Autodesk Inventor part; units mm, degrees
ref_plane "YZ Plane" through (0, 0, 0) normal (1, 0, 0) x (0, 1, 0)
ref_plane "XZ Plane" through (0, 0, 0) normal (0, 1, 0) x (-1, 0, 0)
ref_plane "XY Plane" through (0, 0, 0) normal (0, 0, 1) x (1, 0, 0)
sketch "Sketch2" plane through (0, 0, 0) normal (0, 1, 0) x (-1, 0, 0)
  line L0 (0, 0) -> (-1000, 0)
  line L1 (-1000, 0) -> (-1000, -1000)
  line L2 (-1000, -1000) -> (0, -1000)
  line L3 (0, -1000) -> (0, 0)
  dimension "d0" = 1000
  dimension "d1" = 1000
extrude "Extrusion1" add sketch "Sketch2" along normal blind 1000
shell "Shell1" thickness 30 removed faces 0
sketch "Sketch3" plane through (0, 1000, 0) normal (0, 1, 0) x (1, 0, 0)
  line L0 (30, 30) -> (970, 30)
  line L1 (970, 30) -> (970, 970)
  line L2 (30, 30) -> (970, 30)
  line L3 (970, 30) -> (970, 970)
  line L4 (970, 970) -> (30, 970)
  line L5 (30, 970) -> (30, 30)
  point P0 (0, 0)
extrude "Extrusion2" cut sketch "Sketch3" against normal blind 980
sketch "Sketch4" plane through (1000, 0, -1000) normal (0, 0, -1) x (-1, 0, 0)
  line L0 (30, 20) -> (30, 1000)
  line L1 (30, 30) -> (970, 30)
  line L2 (970, 30) -> (970, 970)
  line L3 (970, 970) -> (30, 970)
  line L4 (30, 970) -> (30, 30)
  line L5 (0, 0) -> (0, 1000)
  line L6 (0, 1000) -> (1000, 1000)
  point P0 (1000, 0)
  point P1 (30, 970)
  dimension "d7" = 940
  dimension "d8" = 940
  dimension "d9" = 30
  dimension "d10" = 30
extrude "Extrusion3" cut sketch "Sketch4" against normal blind 1000
fillet "Fillet1" radius 2 28 edges at (500, 1000, -1000) (500, 1000, 0) (500, 0, -1000) (500, 0, 0) (0, 500, 0) (0, 1000, -500) (0, 500, -1000) (500, 1000, -30) (30, 1000, -500) (500, 1000, -970) (500, 970, -970) (500, 30, -1000) (500, 30, -970) (500, 30, -30) (500, 30, 0) (500, 970, 0) (30, 500, 0) (30, 500, -1000) (0, 0, -500) (1000, 0, -500) (970, 500, 0) (1000, 500, 0) (970, 500, -1000) (1000, 500, -1000) (970, 1000, -500) (1000, 1000, -500) (500, 970, -1000) (30, 20, -500)
sketch "Sketch5" plane through (1000, 2, -2) normal (1, 0, 0) x (0, 0, -1)
  circle A0 centre (500, 500) radius 250
  line L0 (996, 0) -> (0, 0)
  line L1 (0, 0) -> (0, 996)
  point P0 (-2, -2)
  dimension "d14" = 500
  dimension "d15" = 500
  dimension "d16" = 500
extrude "Extrusion4" cut sketch "Sketch5" against normal blind 100
properties part number "Body_prototype2"
Could you check a few things on this model? Use its own coordinates, in mm. A direction names the side the tool comes from. Give positions to 0.01 mm unless a question says otherwise; leave off trailing zeros. Order: outer loops, then holes, each group sorted by start corner. A loop starts at its lowest first (then second) coordinate and runs counter-clockwise, first axis right, second up. Notation, with made-up numbers: M 29.25,60 L 83.25,60 A19 cw 83.25,66 Z; hole C 79,41.5 d4. An arc over 180 degrees is marked long. One line per question, with ' | ' between items.
1. I want a section at A-A (y = 502). List the corners of the cut face in (x, z) for me.
Results:
outline: M 0,-998 A2 ccw 2,-1000 L 28,-1000 A2 ccw 30,-998 L 30,-2 A2 ccw 28,0 L 2,0 A2 ccw 0,-2 Z; M 970,-998 A2 ccw 972,-1000 L 998,-1000 A2 ccw 1000,-998 L 1000,-752 L 970,-752 Z; M 970,-252 L 1000,-252 L 1000,-2 A2 ccw 998,0 L 972,0 A2 ccw 970,-2 Z
2. If I drill on line 1 (X direction, y = 922, z = -222); line 2 (Y direction, x = 992.5, z = -502); line 3 (Y direction, x = 648, z = -812), over which ranges is the centre line in solid material (lowest first)?
Results:
line 1: 0 to 30, 970 to 1000 | line 2: 0 to 252, 752 to 1000 | line 3: 0 to 20
3. I want a section at C-C (x = 550). Give the number of separate pieces and of enclosed holes in the cut face, and give its area (3 significant figures).
Results:
separate pieces: 3 | enclosed holes: 0 | area: 22,400 mm²
4. We'd pull the mould along Y, two halves only. Please class faces 1 (the face through (507, 0, -493)), 2 (the face through (461, 977, 0)), 3 (the face through (985.21, 577.093, -740.455)): +Y half, -Y half, draft (parallel to the pull), parting line (faces both ways), or undercut.
Results:
face 1: -Y half | face 2: draft | face 3: undercut
5. I want a section at B-B (z = -502). List the corners of the cut face in (x, y) for me, and give its area (3 significant figures).
Results:
outline: M 0,2 A2 ccw 2,0 L 998,0 A2 ccw 1000,2 L 1000,252 L 970,252 L 970,20 L 32,20 A2 cw 30,22 L 30,998 A2 ccw 28,1000 L 2,1000 A2 ccw 0,998 Z; M 970,752 L 1000,752 L 1000,998 A2 ccw 998,1000 L 972,1000 A2 ccw 970,998 Z | area: 63,800 mm²
6. I want a section at D-D (y = 822). List the corners of the cut face in (x, z) for me, and give its area (3 significant figures).
Results:
outline: M 0,-998 A2 ccw 2,-1000 L 28,-1000 A2 ccw 30,-998 L 30,-2 A2 ccw 28,0 L 2,0 A2 ccw 0,-2 Z; M 970,-998 A2 ccw 972,-1000 L 998,-1000 A2 ccw 1000,-998 L 1000,-2 A2 ccw 998,0 L 972,0 A2 ccw 970,-2 Z | area: 60,000 mm²
7. For faces 4 (the face through (493, 984, -30)), 5 (the face through (539, 1000, -977)), 6 (the face through (507, 30, -985)), which set-ups out of +Z, -Z, +X, -X, +Y, -Y let a thin tool reach every point of the face, with its end or its side?
Results:
face 4: +Y | face 5: +Z, -Z, +X, -X, +Y | face 6: +Z, -Z
